from build123d import *

# Parameters (mm, degrees)
BOSS_EXTRUDE1_DEPTH = 7
CUT_EXTRUDE1_DEPTH  = 5
SKETCH3_R           = 1.25
CUT_EXTRUDE2_DEPTH  = 8


with BuildPart() as part:
    # Sketch1 → Boss-Extrude1 (new body)
    with BuildSketch(Plane.XY):
        with BuildLine():
            Line((0, 0), (11, 0))
            Line((11, 0), (11, 5))
            Line((11, 5), (0, 5))
            ThreePointArc((0, 5), (-2.5, 2.5), (0, 0))
        make_face()
    extrude(amount=BOSS_EXTRUDE1_DEPTH)

    # Sketch2 → Cut-Extrude1 (cut)
    with BuildSketch(Plane.XY.offset(7)):
        Polygon((11, 3.9), (10.4, 2.5), (9.4, 2.5), (9.1, 3.2), (8.2, 3.2), (7.9, 2.5), (6.9, 2.5), (6.6, 3.2), (5.7, 3.2), (5.4, 2.5), (4.4, 2.5), (4.1, 3.2), (3.2, 3.2), (2.9, 2.5), (1.9, 2.5), (1.9, 1.3), (11, 1.3), align=None)
    extrude(amount=-CUT_EXTRUDE1_DEPTH, mode=Mode.SUBTRACT)

    # Sketch3 → Cut-Extrude2 (cut, through all)
    with BuildSketch(Plane.XY.offset(7)):
        with Locations((0, 2.5)):
            Circle(SKETCH3_R)
    extrude(amount=-CUT_EXTRUDE2_DEPTH, mode=Mode.SUBTRACT)


solid = part.part
Read the model definition and answer for the solid it produces. Units are mm, in the model's axes. A direction names the side the tool comes from. Give positions to 0.01 mm unless a question says otherwise; leave off trailing zeros. Write each loop counter-clockwise with the first axis right and the second up, starting at its lowest first coordinate (ties: lowest second). Pieces come first, ordered by that corner, then holes. Notation, with made-up numbers: (-10, -16) -> (42, -16) arc R20 ccw to (42, -8) -> close; hole circle Ø9 at (-39, 47.25). An arc over 180 degrees is marked (long way). Answer as a JSON object with one key per item and string values. Group by question number.
1) Consider L1, parallel to X at y = 2.6, z = 2.5; L2, parallel to Y at x = 2.5, z = 2.75; L3, parallel to Y at x = 0, z = 2. Determine where each line is inside the solid, lowest interval first. Write a range as from..to.
2) Find section B-B (y = 3.4). Write down the section's boundary in (x, z), and give its area (3 significant figures).
3) The mould has two halves that part along Y. Classify faces 4 (the flat face through (10, 2.5, 5)), 5 (the cylindrical face through (-2.5, 2.6, 3.5)), 6 (the flat face through (4, 4, 7)), 7 (the flat face through (6, 3.2, 5)): +Y half, -Y half, draft (parallel to the pull), parting line (faces both ways), or undercut.
4) Find section D-D (x = -1). Write down the section's boundary in (y, z), and give its area (3 significant figures).
5) This flat-tipped pin is pushed along its axis until it touches: P1, Ø3, axis at y = 0.5, z = 5, coming from the -X side. Where does it stop, or does it pass through?
6) A tool of negligible diameter and unlimited length cuts with its end or side. For faces 1 (the cylindrical face through (-0.16, 3.74, 3.55)), 2 (the flat face through (6, 1.3, 5)), 3 (the flat face through (3.7, 3.2, 4.5)), from which of +Z, -Z, +X, -X, +Y, -Y can it reach the whole face along a straight path? Write none if from no direction.
7) Find section A-A (z = 4.25). Write down the section's boundary in (x, y).
8) Find section C-C (x = 7.25). Write down the section's boundary in (y, z).
Values follow:
{
 "1": {"L1": "x = -2.5..-1.25, 1.25..2.94, 4.36..5.44, 6.86..7.94, 9.36..10.44", "L2": "y = 0..1.3, 2.5..5", "L3": "y = 0..1.25, 3.75..5"},
 "2": {"outline": "(-2.33, 0) -> (-0.87, 0) -> (-0.87, 7) -> (-2.33, 7) -> close; (0.87, 0) -> (11, 0) -> (11, 2) -> (10.79, 2) -> (10.79, 7) -> (0.87, 7) -> close", "area": "80.1 mm2"},
 "3": {"face 4": "undercut", "face 5": "parting line", "face 6": "draft", "face 7": "undercut"},
 "4": {"outline": "(0.21, 0) -> (1.75, 0) -> (1.75, 7) -> (0.21, 7) -> close; (3.25, 0) -> (4.79, 0) -> (4.79, 7) -> (3.25, 7) -> close", "area": "21.6 mm2"},
 "5": {"P1": "stops at x = -2.45"},
 "6": {"face 1": "+Z, -Z", "face 2": "+Z, +X", "face 3": "+Z"},
 "7": {"outline": "(0, 0) -> (11, 0) -> (11, 1.3) -> (1.9, 1.3) -> (1.9, 2.5) -> (2.9, 2.5) -> (3.2, 3.2) -> (4.1, 3.2) -> (4.4, 2.5) -> (5.4, 2.5) -> (5.7, 3.2) -> (6.6, 3.2) -> (6.9, 2.5) -> (7.9, 2.5) -> (8.2, 3.2) -> (9.1, 3.2) -> (9.4, 2.5) -> (10.4, 2.5) -> (11, 3.9) -> (11, 5) -> (0, 5) arc R2.5 ccw to start; hole circle Ø2.5 at (0, 2.5)"},
 "8": {"outline": "(0, 0) -> (5, 0) -> (5, 7) -> (2.5, 7) -> (2.5, 2) -> (1.3, 2) -> (1.3, 7) -> (0, 7) -> close"}
}
